```python
from build123d import *

# Parameters (mm, degrees)
F0_W     = 63.5
F0_H     = 19.05
F1_DEPTH = 381
F2_SIZE  = 3.175
F3_W     = 12.7
F3_H     = 6.35
F4_DEPTH = 381.001
F5_W     = 6.35
F5_H     = 9.525
F6_DEPTH = 50.8


with BuildPart() as f1:
    # F0 (on Top) → F1 (new body)
    with BuildSketch(Plane.XY):
        with Locations((31.75, 9.525)):
            Rectangle(F0_W, F0_H)
    extrude(amount=F1_DEPTH)

    # F2
    f2_edges = [f1.edges().sort_by_distance(p)[0] for p in [
        (0, 0, 190.5),
        (63.5, 0, 190.5),
        (31.75, 0, 381),
        (31.75, 0, 0),
    ]]
    chamfer(f2_edges, length=F2_SIZE)

    # F3 (on face) → F4 (cut, through all)
    with BuildSketch(Plane(origin=(0, 0, 0), x_dir=(1, 0, 0), z_dir=(0, 0, -1))):
        with Locations((57.15, -11.1125)):
            Rectangle(F3_W, F3_H)
    extrude(amount=-F4_DEPTH, mode=Mode.SUBTRACT)

    # F5 (on face) → F6 (join)
    with BuildSketch(Plane(origin=(0, 0, 0), x_dir=(0, -1, 0), z_dir=(-1, 0, 0))):
        with Locations((-11.1125, 385.7625)):
            Rectangle(F5_W, F5_H)
        with Locations((-11.1125, -4.7625)):
            Rectangle(F5_W, F5_H)
    extrude(amount=-F6_DEPTH)


solid = f1.part
```
Can you work these out from the model? Positions are in its coordinate system, mm. A direction names the side the tool comes from. Coordinates: 2 decimals unless noted, no trailing zeros. Loops run counter-clockwise (first coordinate to the right, second up) from the corner with the lowest first, then second, coordinate; pieces in that order, holes last.
1) Thinking about a two-plate mould opening in Y: for faces 1 (the flat face through (31, 19.05, 188)), 2 (the flat face through (31, 0, 188)), 3 (the flat face through (57, 14.288, 188)), which applies, pulls with the +Y half, pulls with the -Y half, needs draft (parallel to the pull), parting line crosses it, or undercut?
2) Imagine slicing it at C-C on y = 11. List the corners of the cut face in (x, z) for me (3 decimals), plus the area to 3 significant figures.
3) I need wall thicknesses on probe 1 along Y at (x, z) = (56, 150); probe 2 along X at (y, z) = (9.5, 280.5); probe 3 along Z at (x, y) = (23, 15). Which ranges of each line are inside material? Lowest first, please.
4) Which directions (+Z, -Z, +X, -X, +Y, -Y) give clear straight access to the entire face, cutting with the end or side of a thin tool? Please do faces 4 (the flat face through (25, 7.938, 386)), 5 (the flat face through (25, 7.938, -5)), 6 (the flat face through (25, 14.288, -5)).
5) For pin 1 (5 mm diameter, centred on x = 42, y = 4.5, fed in from +Z); pin 2 (1.5 mm diameter, centred on x = 14.5, y = 7, fed in from -Z); pin 3 (3 mm diameter, centred on x = 34.5, z = 384, fed in from +Y); pin 4 (10.5 mm diameter, centred on x = 27.5, z = -3.5, fed in from +Y), each with a flat end and sliding along its axis, tell me the tip position at first contact or that it passes through.
Completed:
1. face 1: pulls with the +Y half
1. face 2: pulls with the -Y half
1. face 3: undercut
2. outline: (0, -9.525) - (50.8, -9.525) - (50.8, 390.525) - (0, 390.525) - close
2. area: 20,300 mm2
3. probe 1: y = 0 to 7.94, 14.29 to 19.05
3. probe 2: x = 0 to 50.8
3. probe 3: z = 0 to 381
4. face 4: +Z, +X, -X, -Y
4. face 5: -Z, +X, -X, -Y
4. face 6: -Z, +X, -X, +Y
5. pin 1: stops at z = 381
5. pin 2: stops at z = 0
5. pin 3: stops at y = 14.29
5. pin 4: stops at y = 19.05
